The figure shows three views and two pictorial views of one solid part (mm, origin at its lowest corner). Answer the questions. A direction names the side the tool comes from. Give positions to 0.01 mm unless a question says otherwise; leave off trailing zeros. Order: outer loops, then holes, each group sorted by start corner. A loop starts at its lowest first (then second) coordinate and runs counter-clockwise, first axis right, second up. Notation, with made-up numbers: (23, 81) - (53, 81) arc R29 cw to (53, 101) - close; hole circle Ø1 at (85.25, -9). An arc over 180 degrees is marked (long way). Write item = value, one per line.
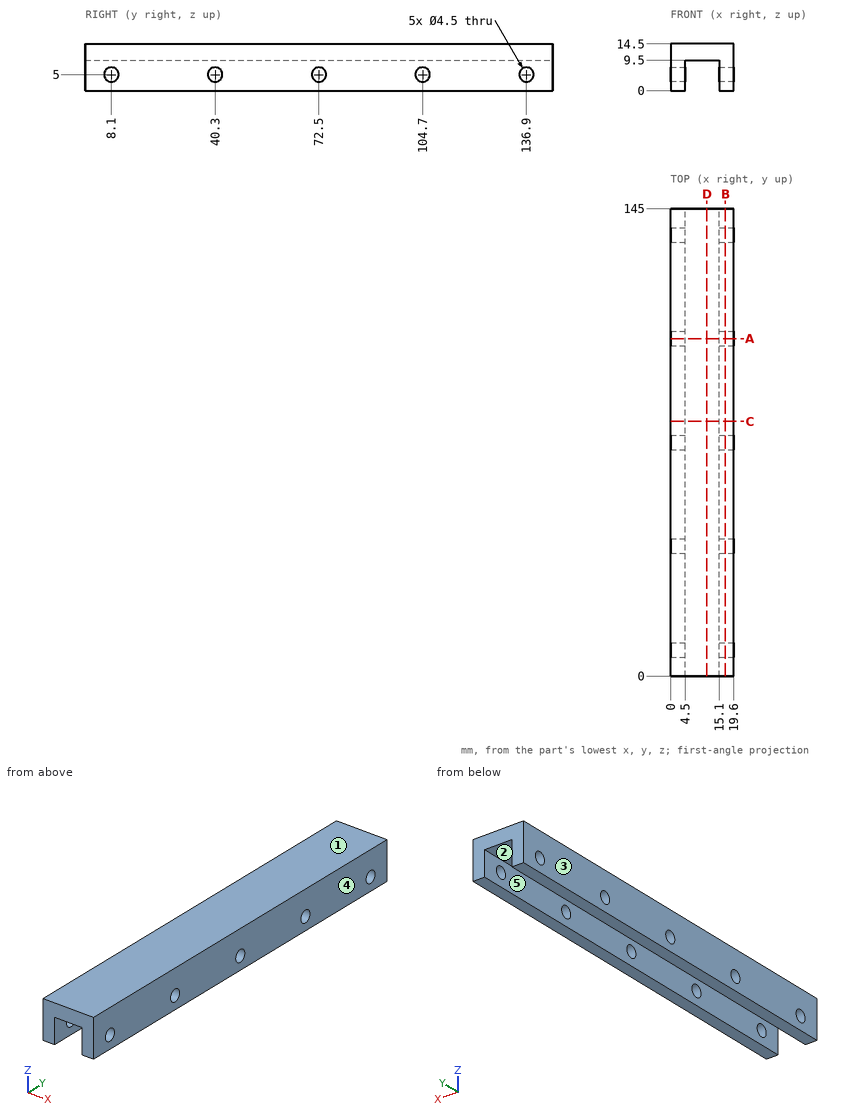
1. Section A-A (y = 104.7) is taken. Determine the outline of the cut face in (x, z).
Recorded:
outline = (0, 0) - (4.5, 0) - (4.5, 2.75) - (0, 2.75) - close; (0, 7.25) - (4.5, 7.25) - (4.5, 9.5) - (15.1, 9.5) - (15.1, 7.25) - (19.6, 7.25) - (19.6, 14.5) - (0, 14.5) - close; (15.1, 0) - (19.6, 0) - (19.6, 2.75) - (15.1, 2.75) - close
2. Section C-C (y = 79) is taken. Determine the outline of the cut face in (x, z).
Recorded:
outline = (0, 0) - (4.5, 0) - (4.5, 9.5) - (15.1, 9.5) - (15.1, 0) - (19.6, 0) - (19.6, 14.5) - (0, 14.5) - close
3. Section B-B (x = 17) is taken. Determine the outline of the cut face in (y, z), and give its area (3 significant figures).
Recorded:
outline = (0, 0) - (145, 0) - (145, 14.5) - (0, 14.5) - close; hole circle Ø4.5 at (8.1, 5); hole circle Ø4.5 at (40.3, 5); hole circle Ø4.5 at (72.5, 5); hole circle Ø4.5 at (104.7, 5); hole circle Ø4.5 at (136.9, 5)
area = 2,020 mm^2
4. Determine the mould class of the marked faces 3, 4 and 5 for opening direction X: +X half, -X half, draft (parallel to the pull), parting line (faces both ways), or undercut.
Recorded:
face_3 = -X half
face_4 = +X half
face_5 = undercut
5. Straight lines are drawn through the part: L1, parallel to Y at x = 16.3, z = 5; L2, parallel to X at y = 131.5, z = 3.75; L3, parallel to Z at x = 13.75, y = 101. For each, find the intervals that lie inside material, in ascending order. Write a range as [from, to].
Recorded:
L1 = [0, 5.85], [10.35, 38.05], [42.55, 70.25], [74.75, 102.45], [106.95, 134.65], [139.15, 145]
L2 = [0, 4.5], [15.1, 19.6]
L3 = [9.5, 14.5]
6. A flat-ended cylindrical pin translates along its axis: pin 1 (4 mm diameter, centred on y = 136.9, z = 5, fed in from +X). Find the tip coordinate at first contact, or state that the pin passes through.
Recorded:
pin_1 = through
7. For the marked faces 1 and 2, determine the directions among +Z, -Z, +X, -X, +Y, -Y from which every point of the face is accessible in a straight line to the end or side of a thin tool.
Recorded:
face_1 = +Z, +X, -X, +Y, -Y
face_2 = -Z, +Y, -Y
8. Section D-D (x = 11.25) is taken. Determine the outline of the cut face in (y, z).
Recorded:
outline = (0, 9.5) - (145, 9.5) - (145, 14.5) - (0, 14.5) - close
